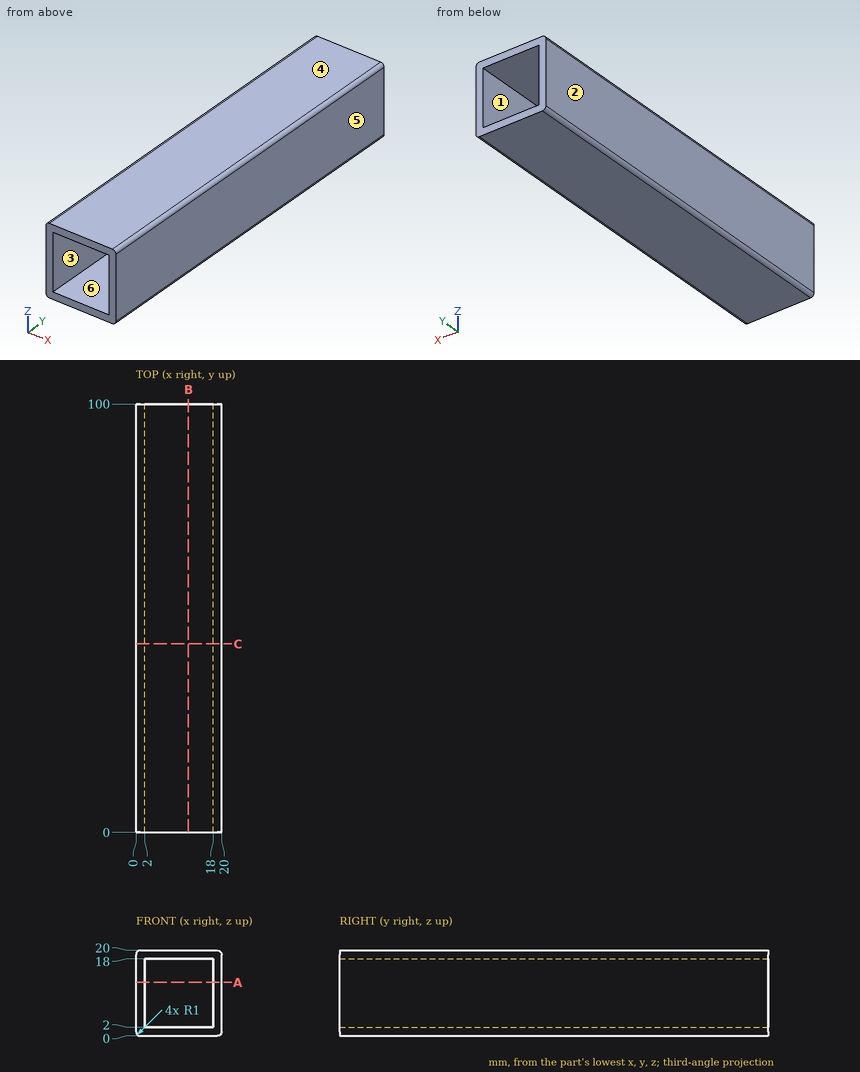
The drawing under review shows one solid part. Ordinate dimensions are in mm from its lowest x, y, z. A direction names the side the tool comes from. Round coordinates to 2 decimals unless told otherwise and drop trailing zeros. Order: outer loops, then holes, each group sorted by start corner. A loop starts at its lowest first (then second) coordinate and runs counter-clockwise, first axis right, second up. Notation, with made-up numbers: (81, -5) -> (120, -5) arc R19 ccw to (120, 20) -> close; hole circle Ø1 at (36, 3). An arc over 180 degrees is marked (long way). Use a Markdown table: item, result.
Q1. Mouldability with a two-part tool opening along Z and no side actions: class the marked faces 3, 4, 5 and 6 as +Z half, -Z half, draft (parallel to the pull), parting line (faces both ways), or undercut.
Values:
| item | result |
|---|---|
| face 3 | undercut |
| face 4 | +Z half |
| face 5 | draft |
| face 6 | undercut |
Q2. We need section B-B on x = 12.25. Write out the cut boundary in (y, z).
Values:
| item | result |
|---|---|
| outline | (0, 0) -> (100, 0) -> (100, 2) -> (0, 2) -> close; (0, 18) -> (100, 18) -> (100, 20) -> (0, 20) -> close |
Q3. We need section C-C on y = 44. Write out the cut boundary in (x, z).
Values:
| item | result |
|---|---|
| outline | (0, 1) arc R1 ccw to (1, 0) -> (19, 0) arc R1 ccw to (20, 1) -> (20, 19) arc R1 ccw to (19, 20) -> (1, 20) arc R1 ccw to (0, 19) -> close; hole (2, 2) -> (18, 2) -> (18, 18) -> (2, 18) -> close |
Q4. Tool access review of the marked faces 1 and 2: name each direction out of +Z, -Z, +X, -X, +Y, -Y from which nothing blocks a thin tool from reaching the whole face with its end or side.
Values:
| item | result |
|---|---|
| face 1 | +Y, -Y |
| face 2 | +Z, -Z, -X, +Y, -Y |
Q5. For line 1 (Z direction, x = 12.75, y = 58.5), list the stretches that pass through material, from the lowest coordinate up.
Values:
| item | result |
|---|---|
| line 1 | z = 0 to 2, 18 to 20 |
Q6. We need section A-A on z = 12.5. Write out the cut boundary in (x, y).
Values:
| item | result |
|---|---|
| outline | (0, 0) -> (2, 0) -> (2, 100) -> (0, 100) -> close; (18, 0) -> (20, 0) -> (20, 100) -> (18, 100) -> close |
